```python
from build123d import *

# Parameters (mm, degrees)
MODEL_W                  = 73.99999408
MODEL_H                  = 173.99998608
MODEL_R                  = 1.5
MODEL_R_2                = 1.799999856
MODEL_R_3                = 1.49999988
MODEL_R_4                = 3.99999968
MODEL_R_5                = 6.2499995
MODEL_W_2                = 40.99999672
MODEL_H_2                = 99.49999204
MODEL_W_3                = 19.999994237
MODEL_H_3                = 6.600001389
RESSALTO_EXTRUS_O1_DEPTH = 6


with BuildPart() as part:
    # Model → Ressalto-extrusão1 (new body)
    with BuildSketch(Plane.XY):
        with Locations((67.822014365, 94.353551358)):
            Rectangle(MODEL_W, MODEL_H)
        with Locations((87.822012765, 21.853557158)):
            Circle(MODEL_R, mode=Mode.SUBTRACT)
        with Locations((49.822015805, 14.131755092)):
            Circle(MODEL_R_2, mode=Mode.SUBTRACT)
        with Locations((37.822016765, 21.853557158)):
            Circle(MODEL_R_3, mode=Mode.SUBTRACT)
        with Locations((87.822012765, 166.853545558)):
            Circle(MODEL_R_3, mode=Mode.SUBTRACT)
        with Locations((81.822013245, 155.853546358)):
            Circle(MODEL_R_4, mode=Mode.SUBTRACT)
        with Locations((64.822014605, 155.853546358)):
            Circle(MODEL_R_4, mode=Mode.SUBTRACT)
        with Locations((45.322016165, 155.853546358)):
            Circle(MODEL_R_5, mode=Mode.SUBTRACT)
        with Locations((37.822016765, 166.853545558)):
            Circle(MODEL_R_3, mode=Mode.SUBTRACT)
        with Locations((49.822015805, 174.808809717)):
            Circle(MODEL_R_2, mode=Mode.SUBTRACT)
        with Locations((68.622014301, 82.103552338)):
            Rectangle(MODEL_W_2, MODEL_H_2, mode=Mode.SUBTRACT)
        with Locations((67.822014365, 14.131755092)):
            Rectangle(MODEL_W_3, MODEL_H_3, mode=Mode.SUBTRACT)
        with Locations((67.822014365, 174.808809717)):
            Rectangle(MODEL_W_3, MODEL_H_3, mode=Mode.SUBTRACT)
    extrude(amount=RESSALTO_EXTRUS_O1_DEPTH)


solid = part.part
```
Geometry check sheet. Reference: the model listing, model coordinates, mm. A direction names the side the tool comes from. Round coordinates to 2 decimals unless told otherwise and drop trailing zeros. Order: outer loops, then holes, each group sorted by start corner. A loop starts at its lowest first (then second) coordinate and runs counter-clockwise, first axis right, second up. Notation, with made-up numbers: M 39,56.5 L 74,56.5 A32 ccw 74,88.5 Z; hole C -0.75,-9.75 d2. An arc over 180 degrees is marked long. Write item = value, one per line.
Q1. Scan lines: line 1 (Y direction, x = 60, z = 4.2); line 2 (Y direction, x = 37.5, z = 0.5); line 3 (Y direction, x = 65, z = 3.1). Record each from-to range of solid material in increasing order.
Answer block:
line_1 = 7.35 to 10.83, 17.43 to 32.35, 131.85 to 171.51, 178.11 to 181.35
line_2 = 7.35 to 20.39, 23.32 to 165.39, 168.32 to 181.35
line_3 = 7.35 to 10.83, 17.43 to 32.35, 131.85 to 151.86, 159.85 to 171.51, 178.11 to 181.35
Q2. Depth check by flat-ended pin: pin 1 Ø4 at (x, y) = (87.82, 21.85) entering from +Z; pin 2 Ø1.8 at (x, y) = (37.82, 166.85) entering from -Z. Enter the tip coordinate at first touch or a pass-through.
Answer block:
pin_1 = 6
pin_2 = through
Q3. Section check B-B (x = 55). Enter the section's corners in (y, z).
Answer block:
outline = M 7.35,0 L 32.35,0 L 32.35,6 L 7.35,6 Z; M 131.85,0 L 181.35,0 L 181.35,6 L 131.85,6 Z
Q4. Set-up check for faces 1 (the flat face through (89.122, 81, 3)), 2 (the flat face through (92, 96, 0)): record each of +Z, -Z, +X, -X, +Y, -Y from which the full face is reachable in a straight line by a thin tool's end or side.
Answer block:
face_1 = +Z, -Z
face_2 = -Z, +X, -X, +Y, -Y
Q5. Release check for a two-part mould opening along Y. For faces 3 (the flat face through (104.822, 93, 3)), 4 (the flat face through (77.822, 14, 3)) record: released by +Y, released by -Y, zero draft, split by the parting line, or undercut.
Answer block:
face_3 = zero draft
face_4 = undercut
Q6. Section check C-C (z = 3.6). Give the number of separate pieces and of enclosed holes in the cut face, plus the area to 3 significant figures.
Answer block:
separate_pieces = 1
enclosed_holes = 12
area = 8,260 mm^2
Q7. Section check A-A (y = 60.5). Enter the section's corners in (x, z), plus the area to 3 significant figures.
Answer block:
outline = M 30.82,0 L 48.12,0 L 48.12,6 L 30.82,6 Z; M 89.12,0 L 104.82,0 L 104.82,6 L 89.12,6 Z
area = 198 mm^2
